Here's how the part is built. I have some questions about the finished solid (model axes, mm). Round coordinates to 2 decimals unless told otherwise and drop trailing zeros. Write each loop counter-clockwise with the first axis right and the second up, starting at its lowest first coordinate (ties: lowest second). Pieces come first, ordered by that corner, then holes. Notation, with made-up numbers: M -12,15 L 16,15 A22 cw 16,30 Z; hole C 53.25,73.5 d5. An arc over 180 degrees is marked long. Use one line per item in the form item = value. Start each with the question number.
Q1. I want a section at A-A on y = 43. List the corners of the cut face in (x, z) for me.
Q2. I'm going to push flat-ended pins straight in: pin 1 Ø1.5 at (x, z) = (-24.5, 1) entering from +Y; pin 2 Ø1 at (x, z) = (-70, 1) entering from +Y. Where does each tip first touch, or does it pass through?
Q3. I want a section at B-B on y = 20. List the corners of the cut face in (x, z) for me, and give its area (3 significant figures).
Q4. I need wall thicknesses on line 1 along Y through (x, z) = (0, 1.7); line 2 along Y through (x, z) = (-60, 1.7); line 3 along Y through (x, z) = (55, 1.85). Which ranges of each line are inside material? Lowest first, please. Write a range as from..to.
Q5. I want a section at C-C on z = 2.45. State how many separate pieces and enclosed holes the cut face has, and give its area (3 significant figures).
```python
from build123d import *

# Parameters (mm, degrees)
SKETCH_1_R      = 4
SKETCH_1_R_2    = 1.5
EXTRUDE_1_DEPTH = 3
FILLET_1_R      = 5
FILLET_2_R      = 5
FILLET_3_R      = 5


with BuildPart() as part:
    # 草图1 → 凸台-拉伸1 (new body)
    with BuildSketch(Plane.XY):
        with BuildLine():
            Line((101.056239558, 66.72819932), (0, 53))
            Line((0, 53), (-101.056239558, 66.72819932))
            Line((-101.056239558, 66.72819932), (-103.05702305, 67))
            ThreePointArc((-103.05702305, 67), (-110.280675742, 61.517137029), (-106.942649005, 53.085024478))
            Line((-106.942649005, 53.085024478), (-5.180834606, -8.553300696))
            ThreePointArc((-5.180834606, -8.553300696), (-3.881694774, -9.215880082), (-2.5, -9.682458366))
            ThreePointArc((-2.5, -9.682458366), (0, -10), (2.5, -9.682458366))
            ThreePointArc((2.5, -9.682458366), (3.881694774, -9.215880082), (5.180834606, -8.553300696))
            Line((5.180834606, -8.553300696), (106.942649005, 53.085024478))
            ThreePointArc((106.942649005, 53.085024478), (110.280675742, 61.517137029), (103.05702305, 67))
            Line((103.05702305, 67), (101.056239558, 66.72819932))
        make_face()
        Circle(SKETCH_1_R, mode=Mode.SUBTRACT)
        with BuildLine():
            Line((-38.470197272, 17.456153435), (-2.5, 47.638732699))
            Line((-2.5, 47.638732699), (-2.5, 9.682458366))
            ThreePointArc((-2.5, 9.682458366), (-7.840929555, 6.206434058), (-9.997792991, 0.210084034))
            Line((-9.997792991, 0.210084034), (-38.470197272, 17.456153435))
        make_face(mode=Mode.SUBTRACT)
        with BuildLine():
            Line((38.470197272, 17.456153435), (9.997792991, 0.210084034))
            ThreePointArc((9.997792991, 0.210084034), (7.840929555, 6.206434058), (2.5, 9.682458366))
            Line((2.5, 9.682458366), (2.5, 47.638732699))
            Line((2.5, 47.638732699), (38.470197272, 17.456153435))
        make_face(mode=Mode.SUBTRACT)
        Polygon((-76.992375251, 58.413267417), (-46.919815599, 22.574186413), (-91.163166243, 49.372903102), (-79.915961764, 58.810428231), align=None, mode=Mode.SUBTRACT)
        Polygon((-69.625606174, 57.412513038), (-8.52297152, 49.111895964), (-40.292213402, 22.454336819), align=None, mode=Mode.SUBTRACT)
        with BuildLine():
            Line((-95.680736217, 52.109248249), (-98.304134778, 53.698271544))
            ThreePointArc((-98.304134778, 53.698271544), (-95.998027486, 56.966113336), (-95.699425849, 60.954566405))
            Line((-95.699425849, 60.954566405), (-86.610723734, 59.719892378))
            Line((-86.610723734, 59.719892378), (-95.680736217, 52.109248249))
        make_face(mode=Mode.SUBTRACT)
        with Locations((-103.05702305, 59.5)):
            Circle(SKETCH_1_R_2, mode=Mode.SUBTRACT)
        Polygon((40.292213402, 22.454336819), (8.52297152, 49.111895964), (69.625606174, 57.412513038), align=None, mode=Mode.SUBTRACT)
        Polygon((91.163166243, 49.372903102), (46.919815599, 22.574186413), (76.992375251, 58.413267417), (79.915961764, 58.810428231), align=None, mode=Mode.SUBTRACT)
        with BuildLine():
            Line((95.680736217, 52.109248249), (86.610723734, 59.719892378))
            Line((86.610723734, 59.719892378), (95.699425849, 60.954566405))
            ThreePointArc((95.699425849, 60.954566405), (95.998027486, 56.966113336), (98.304134778, 53.698271544))
            Line((98.304134778, 53.698271544), (95.680736217, 52.109248249))
        make_face(mode=Mode.SUBTRACT)
        with Locations((103.05702305, 59.5)):
            Circle(SKETCH_1_R_2, mode=Mode.SUBTRACT)
    extrude(amount=EXTRUDE_1_DEPTH)

    # 圆角1
    # the kernel refuses this fillet: 5 mm, written as the material it adds along each edge
    with BuildSketch(Plane(origin=(76.992375251, 58.413267417, 0), x_dir=(0.9908985592379703, 0.1346107176272178, 0), z_dir=(0, 0, 1))) as fillet_1_piece_1:
        with BuildLine():
            CenterArc((FILLET_1_R * 0.386508582556, -FILLET_1_R), FILLET_1_R, 90, 42.263889815)
            Line((-FILLET_1_R * 0.286037651021, -FILLET_1_R * 0.259944891443), (0, 0))
            Line((0, 0), (FILLET_1_R * 0.386508582556, 0))
        make_face()
    extrude(amount=3)
    with BuildSketch(Plane(origin=(79.915961764, 58.810428231, 0), x_dir=(0.7660444431189772, -0.6427876096865403, 0), z_dir=(0, 0, 1))) as fillet_1_piece_2:
        with BuildLine():
            CenterArc((FILLET_1_R * 0.442472138408, -FILLET_1_R), FILLET_1_R, 90, 47.736110185)
            Line((-FILLET_1_R * 0.297582970149, -FILLET_1_R * 0.327453766423), (0, 0))
            Line((0, 0), (FILLET_1_R * 0.442472138408, 0))
        make_face()
    extrude(amount=3)

    # 圆角2
    # the kernel refuses this fillet: 5 mm, written as the material it adds along each edge
    with BuildSketch(Plane(origin=(-79.915961764, 58.810428231, 0), x_dir=(0.9908985592379704, -0.13461071762721746, 0), z_dir=(0, 0, 1))) as fillet_2_piece_1:
        with BuildLine():
            CenterArc((FILLET_2_R * 0.442472138408, -FILLET_2_R), FILLET_2_R, 90, 47.736110185)
            Line((-FILLET_2_R * 0.297582970149, -FILLET_2_R * 0.327453766423), (0, 0))
            Line((0, 0), (FILLET_2_R * 0.442472138408, 0))
        make_face()
    extrude(amount=3)
    with BuildSketch(Plane(origin=(-76.992375251, 58.413267417, 0), x_dir=(0.642787609686538, -0.7660444431189791, 0), z_dir=(0, 0, 1))) as fillet_2_piece_2:
        with BuildLine():
            CenterArc((FILLET_2_R * 0.386508582556, -FILLET_2_R), FILLET_2_R, 90, 42.263889815)
            Line((-FILLET_2_R * 0.286037651021, -FILLET_2_R * 0.259944891443), (0, 0))
            Line((0, 0), (FILLET_2_R * 0.386508582556, 0))
        make_face()
    extrude(amount=3)

    # 圆角3
    fillet_3_edges = [part.edges().sort_by_distance(p)[0] for p in [
        (-2.5, 9.682458366, 1.5),
        (2.5, 9.682458366, 1.5),
    ]]
    fillet(fillet_3_edges, radius=FILLET_3_R)


solid = part.part
```
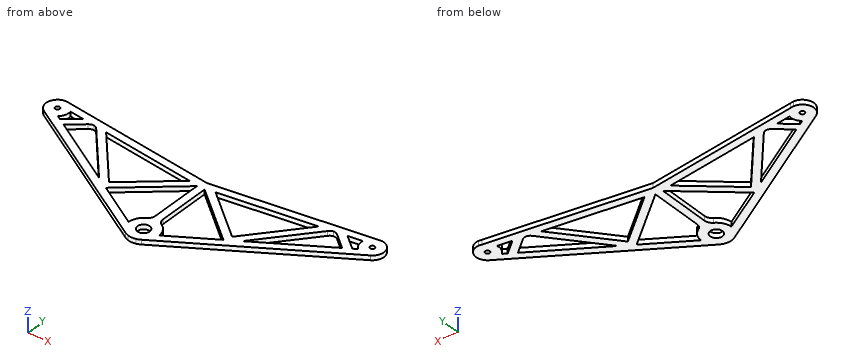
Reported:
q1.outline = M -90.29,0 L -80.64,0 L -80.64,3 L -90.29,3 Z; M -64.06,0 L -57.53,0 L -57.53,3 L -64.06,3 Z; M -15.81,0 L -8.03,0 L -8.03,3 L -15.81,3 Z; M -2.5,0 L 2.5,0 L 2.5,3 L -2.5,3 Z; M 8.03,0 L 15.81,0 L 15.81,3 L 8.03,3 Z; M 57.53,0 L 64.06,0 L 64.06,3 L 57.53,3 Z; M 80.64,0 L 90.29,0 L 90.29,3 L 80.64,3 Z
q2.pin_1 = 56.43
q2.pin_2 = 62.58
q3.outline = M -52.32,0 L -35.44,0 L -35.44,3 L -52.32,3 Z; M -2.5,0 L 2.5,0 L 2.5,3 L -2.5,3 Z; M 35.44,0 L 52.32,0 L 52.32,3 L 35.44,3 Z
q3.area = 116 mm^2
q4.line_1 = -10..-4, 4..53
q4.line_2 = 24.65..30.5, 38.16..45.94, 56.1..61.15
q4.line_3 = 21.62..27.47, 32.2..39.98, 55.43..60.47
q5.separate_pieces = 1
q5.enclosed_holes = 11
q5.area = 3,930 mm^2
